Solid Edge part; units mm, degrees
sketch "Sketch1" plane through (0, 0, 0) normal (0, 0, 1) x (1, 0, 0)
  line L0 (-150, -100) -> (150, -100)
  line L1 (150, -100) -> (150, 100)
  line L2 (150, 100) -> (-150, 100)
  line L3 (-150, 100) -> (-150, -100)
  dimension "D1" = 150
  dimension "D2" = 150
extrude "Protrusion1" add sketch "Sketch1" along normal blind 5
sketch "Sketch2" plane through (0, 0, 5) normal (0, 0, 1) x (1, 0, 0)
  line L0 (-120, -80) -> (-70, -80)
  line L1 (-70, -80) -> (-70, -60)
  line L2 (-70, -60) -> (-120, -60)
  line L3 (-120, -60) -> (-120, -80)
  dimension "D1" = 120
  dimension "D2" = 70
  dimension "D3" = 70
extrude "Cutout1" cut sketch "Sketch2" against normal up to next
sketch "Sketch3" plane through (0, 0, 5) normal (0, 0, 1) x (1, 0, 0)
  line L0 (-145, -95) -> (145, -95)
  line L1 (145, -95) -> (145, 95)
  line L2 (145, 95) -> (-145, 95)
  line L3 (-145, 95) -> (-145, -95)
  line L4 (-150, -100) -> (150, -100)
  line L5 (150, -100) -> (150, 100)
  line L6 (150, 100) -> (-150, 100)
  line L7 (-150, 100) -> (-150, -100)
extrude "ExtrudedProtrusion_2" add sketch "Sketch3" along normal blind 25
sketch "Sketch4" plane through (-150, 0, 15) normal (-1, 0, 0) x (0, -1, 0)
  line L0 (-30, -10) -> (10, -10)
  line L1 (10, -10) -> (10, 5)
  line L2 (10, 5) -> (-30, 5)
  line L3 (-30, 5) -> (-30, -10)
  dimension "D1" = 10
  dimension "D2" = 10
extrude "ExtrudedCutout_2" cut sketch "Sketch4" against normal blind 5
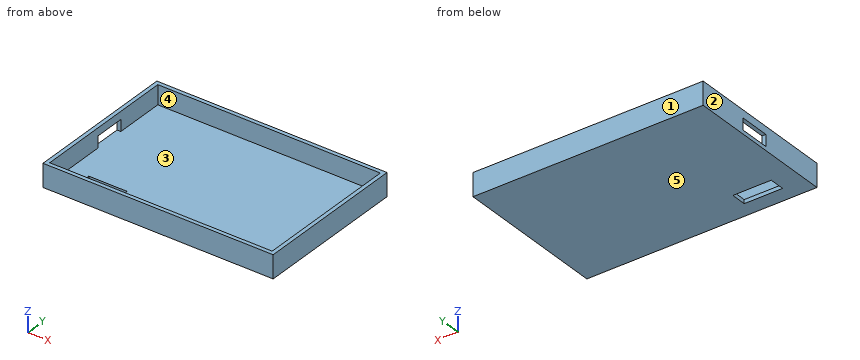
Check sheet for the modelled part. Datum: model origin and axes. Units: mm. Face numbers are marked on the shaded views. A direction names the side the tool comes from. Coordinates: 2 decimals unless noted, no trailing zeros. Write each loop counter-clockwise with the first axis right and the second up, starting at its lowest first coordinate (ties: lowest second). Pieces come first, ordered by that corner, then holes. Notation, with made-up numbers: M -5,-17.5 L 51,-17.5 A17 cw 51,10.5 Z; hole C -40,31.5 d4. An arc over 180 degrees is marked long. Write item = value, one per line. Start each with the question number.
1. Mould release check, pull along Y, two halves, no side actions. Record for the marked faces 1, 2 and 3: pulls with the +Y half, pulls with the -Y half, needs draft (parallel to the pull), parting line crosses it, or undercut.
2. Sectioned sample at D-D (x = 132). Record the cut outline in (y, z), then the cut area to 3 significant figures.
3. Sectioned sample at C-C (y = 80). Record the cut outline in (x, z).
4. Sectioned sample at A-A (z = 25). Record the cut outline in (x, y).
5. Sectioned sample at B-B (x = -113). Record the cut outline in (y, z), then the cut area to 3 significant figures.
6. Go/stop test with flat-tipped pins: pin 1 (12.5 mm diameter, centred on y = 2, z = 11.5, fed in from -X); pin 2 (12 mm diameter, centred on x = -92.5, y = -43.5, fed in from +Z). Record where each tip stops, or that it passes through.
7. Thickness scan on probe 1 along Y at (x, z) = (3.5, 26.75); probe 2 along X at (y, z) = (-21.5, 19); probe 3 along Z at (x, y) = (51, -1). Record the ranges inside material, lowest first.
8. Tool access check on the marked faces 4 and 5. Record the directions out of +Z, -Z, +X, -X, +Y, -Y that give a thin tool (end or side, any length) a straight path to the whole face; none if there is none.
The answers:
q1.face_1 = pulls with the +Y half
q1.face_2 = needs draft
q1.face_3 = undercut
q2.outline = M -100,0 L 100,0 L 100,30 L 95,30 L 95,5 L -95,5 L -95,30 L -100,30 Z
q2.area = 1,250 mm²
q3.outline = M -150,0 L 150,0 L 150,30 L 145,30 L 145,5 L -145,5 L -145,30 L -150,30 Z
q4.outline = M -150,-100 L 150,-100 L 150,100 L -150,100 Z; hole M -145,-95 L 145,-95 L 145,95 L -145,95 Z
q5.outline = M -100,0 L -80,0 L -80,5 L -95,5 L -95,30 L -100,30 Z; M -60,0 L 100,0 L 100,30 L 95,30 L 95,5 L -60,5 Z
q5.area = 1,150 mm²
q6.pin_1 = 145
q6.pin_2 = 5
q7.probe_1 = -100 to -95, 95 to 100
q7.probe_2 = -150 to -145, 145 to 150
q7.probe_3 = 0 to 5
q8.face_4 = +Z
q8.face_5 = -Z, +X, -X, +Y, -Y
